Verification items for the finished model (mm, model axes). Face numbers are marked on the shaded views. A direction names the side the tool comes from. Coordinates: 2 decimals unless noted, no trailing zeros. Order: outer loops, then holes, each group sorted by start corner. A loop starts at its lowest first (then second) coordinate and runs counter-clockwise, first axis right, second up. Notation, with made-up numbers: M 22,57 L 50,57 A10 ccw 50,65 Z; hole C 75,65 d11. An arc over 180 degrees is marked long. Return JSON: item names as keys, results as strings. Group by question number.
Q1. Thickness scan on probe 1 along Z at (x, y) = (12.5, -7) (3 decimals); probe 2 along Y at (x, z) = (-8.5, 5); probe 3 along Y at (x, z) = (-10, 6). Record the ranges inside material, lowest first.
Q2. Mould release check, pull along Y, two halves, no side actions. Record for the marked faces 4, 5 and 6: pulls with the +Y half, pulls with the -Y half, needs draft (parallel to the pull), parting line crosses it, or undercut.
Q3. Access from +Z, -Z, +X, -X, +Y, -Y to the whole of each face (thin tool, end or side, straight path). Record for the marked faces 1, 2 and 3.
Q4. Section check C-C, the plane z = -11.5. Enter the section's corners in (x, y) (3 decimals).
Q5. Go/stop test with flat-tipped pins: pin 1 Ø8 at (y, z) = (2.5, -15) entering from -X; pin 2 Ø5 at (y, z) = (23.5, -14) entering from -X; pin 3 Ø5 at (x, z) = (21.5, -11) entering from -Y. Record where each tip stops, or that it passes through.
Q6. Section check A-A, the plane x = -1. Enter the section's corners in (y, z) (3 decimals).
Q7. Section check B-B, the plane y = 2.5. Enter the section's corners in (x, z) (3 decimals).
Q8. Section check D-D, the plane x = -7.5. Enter the section's corners in (y, z) (3 decimals), then the cut area to 3 significant figures.
from build123d import *

# Parameters (mm, degrees)
SKETCH1_R           = 11.1
BOSS_EXTRUDE5_DEPTH = 9.525
BOSS_EXTRUDE6_DEPTH = 25


with BuildPart() as part:
    # Sketch1 → Boss-Extrude5 (new body)
    with BuildSketch(Plane.XY):
        with BuildLine():
            ThreePointArc((0, 19.051378432), (-13.47135888, -13.47135888), (19.051378432, 0))
            Line((19.051378432, 0), (28.575, 0))
            ThreePointArc((28.575, 0), (20.205576272, 20.205576272), (0, 28.575))
            Line((0, 28.575), (0, 19.051378432))
        make_face()
        with Locations(Location((0, 0, 0), (0, 0, 180))):
            Circle(SKETCH1_R, mode=Mode.SUBTRACT)
    extrude(amount=BOSS_EXTRUDE5_DEPTH)

    # Sketch2 → Boss-Extrude6 (add)
    with BuildSketch(Plane(origin=(0, 0, 0), x_dir=(-1, 0, 0), z_dir=(0, 0, -1))):
        with BuildLine():
            add(Edge.make_bspline(
                [(0, 28.575), (-21.908651484, 21.908651484), (-28.575, 0)],
                knots=[0, 0, 0, 1, 1, 1], degree=2))
            ThreePointArc((-28.575, 0), (-20.205576272, 20.205576272), (0, 28.575))
        make_face()
        with BuildLine():
            Line((0, 19.4), (0, 28.575))
            add(Edge.make_bspline(
                [(0, 28.575), (-21.908651484, 21.908651484), (-28.575, 0)],
                knots=[0, 0, 0, 1, 1, 1], degree=2))
            Line((-28.575, 0), (-19.4, 0))
            ThreePointArc((-19.4, 0), (-13.717871555, 13.717871555), (0, 19.4))
        make_face()
    extrude(amount=BOSS_EXTRUDE6_DEPTH)


solid = part.part
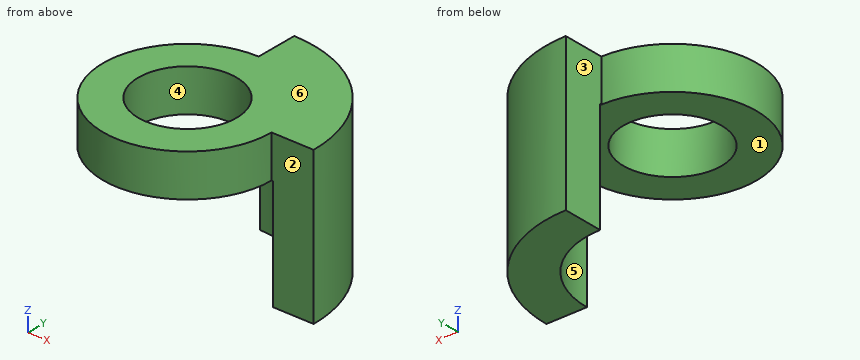
Numbers:
{
 "1": {"probe 1": "z = 0 to 9.525", "probe 2": "y = -17.05 to -7.14, 7.14 to 17.05", "probe 3": "y = -16.22 to -4.82, 4.82 to 16.22"},
 "2": {"face 4": "undercut", "face 5": "pulls with the -Y half", "face 6": "needs draft"},
 "3": {"face 1": "-Z, -X, -Y", "face 2": "+Z, -Z, +X, -Y", "face 3": "+Z, -Z, -X, +Y"},
 "4": {"outline": "M 0,19.4 A19.4 cw 19.4,0 L 28.575,0 A28.575 ccw 0,28.575 Z"},
 "5": {"pin 1": "stops at x = 18.28", "pin 2": "stops at x = 0", "pin 3": "stops at y = 0"},
 "6": {"outline": "M -19.025,0 L -11.055,0 L -11.055,9.525 L -19.025,9.525 Z; M 11.055,0 L 19.025,0 L 19.025,9.525 L 11.055,9.525 Z"},
 "7": {"outline": "M -18.887,0 L -10.815,0 L -10.815,9.525 L -18.887,9.525 Z; M 10.815,0 L 19.238,0 L 19.238,-25 L 28.465,-25 L 28.465,9.525 L 10.815,9.525 Z"},
 "8": {"outline": "M -17.513,0 L -8.183,0 L -8.183,9.525 L -17.513,9.525 Z; M 8.183,0 L 17.513,0 L 17.513,9.525 L 8.183,9.525 Z", "area": "178 mm2"}
}
